CAD build for the part. Positions are in the model's coordinates, mm. Coordinates: 2 decimals unless noted, no trailing zeros. Order: outer loops, then holes, each group sorted by start corner. A loop starts at its lowest first (then second) coordinate and runs counter-clockwise, first axis right, second up. Notation, with made-up numbers: (-0.5, -24) - (40.5, -24) arc R20 ccw to (40.5, 5) - close; hole circle Ø9 at (42.25, -9). An arc over 180 degrees is marked (long way). Use one line per item in the form item = value.
```python
from build123d import *

# Parameters (mm, degrees)
CROQUIS1_R              = 100
CROQUIS1_R_2            = 1.65
CROQUIS1_R_3            = 3.175
CROQUIS1_R_4            = 1.559752628
SALIENTE_EXTRUIR1_DEPTH = 3


with BuildPart() as part:
    # Croquis1 → Saliente-Extruir1 (new body)
    with BuildSketch(Plane(origin=(0, 0, 0), x_dir=(1, 0, 0), z_dir=(0, 1, 0))):
        with Locations(Location((0, 0, 0), (0, 0, 270))):
            Circle(CROQUIS1_R)
        with Locations(Location((40, -85, 0), (0, 0, 270))):
            Circle(CROQUIS1_R_2, mode=Mode.SUBTRACT)
        with Locations(Location((40, 85, 0), (0, 0, 90))):
            Circle(CROQUIS1_R_2, mode=Mode.SUBTRACT)
        with Locations(Location((-40, -85, 0), (0, 0, 90))):
            Circle(CROQUIS1_R_2, mode=Mode.SUBTRACT)
        with Locations(Location((-40, 85, 0), (0, 0, 270))):
            Circle(CROQUIS1_R_2, mode=Mode.SUBTRACT)
        with Locations(Location((-40, 41, 0), (0, 0, 270))):
            Circle(CROQUIS1_R_2, mode=Mode.SUBTRACT)
        with Locations(Location((-40, -41, 0), (0, 0, 270))):
            Circle(CROQUIS1_R_2, mode=Mode.SUBTRACT)
        with Locations(Location((-24, 0, 0), (0, 0, 270))):
            Circle(CROQUIS1_R_3, mode=Mode.SUBTRACT)
        with Locations(Location((-8, 41, 0), (0, 0, 270))):
            Circle(CROQUIS1_R_2, mode=Mode.SUBTRACT)
        with Locations(Location((-8, -41, 0), (0, 0, 270))):
            Circle(CROQUIS1_R_2, mode=Mode.SUBTRACT)
        with Locations(Location((85.070235004, 13.824441517, 0), (0, 0, 270))):
            Circle(CROQUIS1_R_2, mode=Mode.SUBTRACT)
        with Locations(Location((85.070235004, -13.375558483, 0), (0, 0, 270))):
            Circle(CROQUIS1_R_2, mode=Mode.SUBTRACT)
        with Locations(Location((-54.227480628, 72.528357265, 0), (0, 0, 270))):
            Circle(CROQUIS1_R_2, mode=Mode.SUBTRACT)
        with Locations(Location((-62.456735614, 46.603092322, 0), (0, 0, 270))):
            Circle(CROQUIS1_R_4, mode=Mode.SUBTRACT)
        with Locations(Location((-78.396993978, 13.752324836, 0), (0, 0, 270))):
            Circle(CROQUIS1_R_2, mode=Mode.SUBTRACT)
        with Locations(Location((-78.396993978, -13.447675164, 0), (0, 0, 270))):
            Circle(CROQUIS1_R_2, mode=Mode.SUBTRACT)
        with Locations(Location((-65.278300678, -46.636121303, 0), (0, 0, 270))):
            Circle(CROQUIS1_R_2, mode=Mode.SUBTRACT)
        with Locations(Location((-58.238422651, -72.909303778, 0), (0, 0, 270))):
            Circle(CROQUIS1_R_2, mode=Mode.SUBTRACT)
        with BuildLine():
            Line((-51.095611493, -39.959459006), (-43.33104014, -68.937233795))
            ThreePointArc((-43.33104014, -68.937233795), (-46.866574046, -75.060958152), (-52.990298403, -71.525424246))
            Line((-52.990298403, -71.525424246), (-60.754869756, -42.547649457))
            ThreePointArc((-60.754869756, -42.547649457), (-57.21933585, -36.4239251), (-51.095611493, -39.959459006))
        make_face(mode=Mode.SUBTRACT)
        with BuildLine():
            Line((-61.754274717, 15.577653458), (-61.754274717, -14.422346542))
            ThreePointArc((-61.754274717, -14.422346542), (-66.754274717, -19.422346542), (-71.754274717, -14.422346542))
            Line((-71.754274717, -14.422346542), (-71.754274717, 15.577653458))
            ThreePointArc((-71.754274717, 15.577653458), (-66.754274717, 20.577653458), (-61.754274717, 15.577653458))
        make_face(mode=Mode.SUBTRACT)
        with BuildLine():
            Line((-39.917801293, 67.733415285), (-48.810516369, 39.081720421))
            ThreePointArc((-48.810516369, 39.081720421), (-55.067918025, 35.788557123), (-58.361081323, 42.04595878))
            Line((-58.361081323, 42.04595878), (-49.468366247, 70.697653644))
            ThreePointArc((-49.468366247, 70.697653644), (-43.210964591, 73.990816942), (-39.917801293, 67.733415285))
        make_face(mode=Mode.SUBTRACT)
        with BuildLine():
            Line((75.337806397, 15.02279383), (75.337806397, -14.97720617))
            ThreePointArc((75.337806397, -14.97720617), (70.337806397, -19.97720617), (65.337806397, -14.97720617))
            Line((65.337806397, -14.97720617), (65.337806397, 15.02279383))
            ThreePointArc((65.337806397, 15.02279383), (70.337806397, 20.02279383), (75.337806397, 15.02279383))
        make_face(mode=Mode.SUBTRACT)
    extrude(amount=SALIENTE_EXTRUIR1_DEPTH)


solid = part.part
```
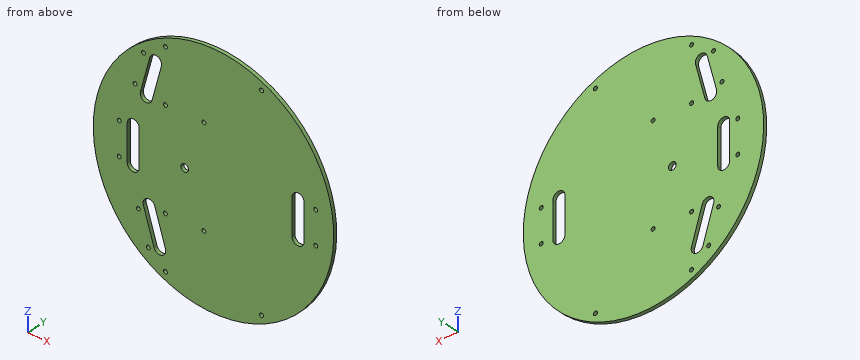
Item 1: Cut at C-C, the plane z = -55. Write the cut outline in (x, y), plus the area to 3 significant figures.
Derived:
outline = (-83.52, 0) - (-54.34, 0) - (-54.34, 3) - (-83.52, 3) - close; (-43.87, 0) - (83.52, 0) - (83.52, 3) - (-43.87, 3) - close
area = 470 mm²
Item 2: Cut at D-D, the plane y = 2.45. State how many separate pieces and enclosed holes the cut face has, plus the area to 3 significant figures.
Derived:
separate_pieces = 1
enclosed_holes = 21
area = 29,700 mm²
Item 3: Cut at B-B, the plane x = -24. Write the cut outline in (y, z) (3 decimals), plus the area to 3 significant figures.
Derived:
outline = (0, -97.077) - (3, -97.077) - (3, -3.175) - (0, -3.175) - close; (0, 3.175) - (3, 3.175) - (3, 97.077) - (0, 97.077) - close
area = 563 mm²
Item 4: Cut at A-A, the plane z = 0. Write the cut outline in (x, y) (3 decimals).
Derived:
outline = (-100, 0) - (-71.754, 0) - (-71.754, 3) - (-100, 3) - close; (-61.754, 0) - (-27.175, 0) - (-27.175, 3) - (-61.754, 3) - close; (-20.825, 0) - (65.338, 0) - (65.338, 3) - (-20.825, 3) - close; (75.338, 0) - (100, 0) - (100, 3) - (75.338, 3) - close
Item 5: Drill centre lines: line 1 (X direction, y = 2, z = 41); line 2 (X direction, y = 0.65, z = -41); line 3 (X direction, y = 2.25, z = -85). Where is each one in solid material? Low to high. Write a range as [from, to].
Derived:
line_1 = [-91.21, -60.92], [-50.82, -41.65], [-38.35, -9.65], [-6.35, 91.21]
line_2 = [-91.21, -58.57], [-48.22, -41.65], [-38.35, -9.65], [-6.35, 91.21]
line_3 = [-52.68, -41.65], [-38.35, 38.35], [41.65, 52.68]
Item 6: Drop flat-ended pins along their axis: pin 1 (4 mm diameter, centred on x = -40, z = 85, fed in from -Y); pin 2 (2 mm diameter, centred on x = -58.24, z = 72.91, fed in from +Y); pin 3 (1.5 mm diameter, centred on y = 2, z = 4.5, fed in from +X). Give the stop position or say it passes through.
Derived:
pin_1 = 0
pin_2 = through
pin_3 = 99.93
